Autodesk Fusion 360 part; units mm, degrees
sketch "Sketch1" plane through (0, 0, 0) normal (0, 0, 1) x (1, 0, 0)
  line L0 (0, 0) -> (-65, 0)
  line L1 (-65, 0) -> (-65, 65)
  line L2 (-65, 65) -> (0, 65)
  line L3 (0, 65) -> (0, 0)
  dimension "d1" = 65
  dimension "d2" = 65
extrude "Extrude1" add sketch "Sketch1" along normal blind 25
sketch "Sketch2" plane through (0, 0, 25) normal (0, 0, 1) x (-1, 0, 0)
  line L0 (0, -65) -> (65, -65)
  line L1 (65, -65) -> (65, 0)
  line L2 (65, 0) -> (0, 0)
  line L3 (0, 0) -> (0, -65)
  line L4 (0, 0) -> (65, 0)
  line L5 (65, 0) -> (65, -7)
  line L6 (65, -7) -> (0, -7)
  line L7 (0, -7) -> (0, 0)
  line L8 (0, 0) -> (7, 0)
  line L9 (7, 0) -> (7, -65)
  line L10 (7, -65) -> (0, -65)
  line L11 (0, -65) -> (0, 0)
  dimension "d5" = 65
  dimension "d6" = 7
  dimension "d7" = 7
fillet "Fillet1" radius 7 1 edges at (-65, 0, 12.5)
fillet "Fillet2" radius 7 1 edges at (0, 65, 12.5)
fillet "Fillet3" radius 7 1 edges at (-65, 65, 12.5)
extrude "Extrude2" cut sketch "Sketch2" against normal blind 3 contours L0 L1 L6 L9
sketch "Sketch3" plane through (0, 0, 22) normal (0, 0, 1) x (-1, 0, 0)
  arc A0 (58, -65) -> (65, -58) centre (58, -58) ccw
  line L0 (65, -58) -> (65, -7)
  line L1 (65, -7) -> (7, -7)
  line L2 (7, -7) -> (7, -65)
  line L3 (7, -65) -> (58, -65)
  circle A1 centre (7, -7) radius 5
  dimension "d13" = 10
extrude "Extrude3" cut sketch "Sketch3" along normal blind 3 contours L1 L2 A1 | L1 L2 A1
sketch "Sketch4" plane through (0, 65, 0) normal (0, 1, 0) x (-1, 0, 0)
  line L0 (58, 22) -> (7, 22)
  line L1 (7, 22) -> (7, 0)
  line L2 (7, 0) -> (58, 0)
  line L3 (58, 0) -> (58, 22)
  circle A0 centre (32.6873, 10.9427) radius 2
  dimension "d16" = 4
extrude "Extrude4" cut sketch "Sketch4" against normal blind 25 contours A0
Read the model definition and answer for the solid it produces. Units are mm, in the model's axes. A direction names the side the tool comes from. Round coordinates to 2 decimals unless told otherwise and drop trailing zeros. Loops run counter-clockwise (first coordinate to the right, second up) from the corner with the lowest first, then second, coordinate; pieces in that order, holes last.
Q1. Consider probe 1 along X at (y, z) = (50, 10.75); probe 2 along Z at (x, y) = (-60, 14); probe 3 along Z at (x, y) = (-32.5, 44). Determine where each line is inside the solid, lowest interval first.
Q2. Section D-D on x = -3.5 is taken. Write down the section's boundary in (y, z), and give its area (3 significant figures).
Q3. Which of the six approach directions +Z, -Z, +X, -X, +Y, -Y give full straight-line access (tool end or side, diameter ignored) to faces 4 (the face through (-39, 7, 24)), 5 (the face through (-65, 32, 11)), 6 (the face through (-33, 40, 11))?
Q4. Determine the mould class of faces 1 (the face through (-3, 4, 23)), 2 (the face through (-33, 65, 8)), 3 (the face through (-63, 2.1, 12.7)) for opening direction Y: released by +Y, released by -Y, zero draft, split by the parting line, or undercut.
Q5. Section A-A on x = -17.5 is taken. Write down the section's boundary in (y, z).
Q6. Section B-B on y = 59 is taken. Write down the section's boundary in (x, z).
Q7. Each of these flat-tipped pins is pushed along its axis until it touches: pin 1 (6 mm diameter, centred on x = -7, y = 7, fed in from +Z); pin 2 (2.5 mm diameter, centred on x = -41.5, z = 24, fed in from +Y); pin 3 (2.5 mm diameter, centred on y = 40, z = 23.5, fed in from -X). Where does it stop, or does it pass through?
Q8. Section C-C on y = 47 is taken. Write down the section's boundary in (x, z), and give its area (3 significant figures).
Output:
1. probe 1: x = -65 to -34.68, -30.7 to 0
1. probe 2: z = 0 to 22
1. probe 3: z = 0 to 8.95, 12.93 to 22
2. outline: (0, 0) - (64.06, 0) - (64.06, 25) - (10.57, 25) - (10.57, 22) - (3.43, 22) - (3.43, 25) - (0, 25) - close
2. area: 1,580 mm2
3. face 4: +Z, -X, +Y
3. face 5: +Z, -Z, -X, +Y, -Y
3. face 6: +Y
4. face 1: undercut
4. face 2: released by +Y
4. face 3: released by -Y
5. outline: (0, 0) - (65, 0) - (65, 22) - (7, 22) - (7, 25) - (0, 25) - close
6. outline: (-64.93, 0) - (-0.07, 0) - (-0.07, 25) - (-7, 25) - (-7, 22) - (-64.93, 22) - close; hole circle Ø4 at (-32.69, 10.94)
7. pin 1: stops at z = 22
7. pin 2: stops at y = 7
7. pin 3: stops at x = -7
8. outline: (-65, 0) - (0, 0) - (0, 25) - (-7, 25) - (-7, 22) - (-65, 22) - close; hole circle Ø4 at (-32.69, 10.94)
8. area: 1,440 mm2
